Input: part model. Units: mm. Frame: model coordinates. Face numbers are marked on the shaded views. A direction names the side the tool comes from. Give positions to 0.01 mm unless a question says otherwise; leave off trailing zeros. Order: outer loops, then holes, each group sorted by start corner. A loop starts at its lowest first (then second) coordinate and runs counter-clockwise, first axis right, second up. Notation, with made-up numbers: (26.25, 72.25) - (82.25, 72.25) arc R24 cw to (82.25, 111.25) - close; hole circle Ø4 at (40.25, 83). An arc over 180 degrees is marked (long way). Use a Markdown table: item, result.
from build123d import *

# Parameters (mm, degrees)
F0_W        = 105
F0_H        = 23
F1_DEPTH    = 6.35
F2_W        = 72
F2_H        = 10
F3_DEPTH    = 25.4
F4_R        = 2.9337
F5_DEPTH    = 25.4
F6_T1_DEPTH = 6.35
F7_W        = 105
F7_H        = 23
F7_R        = 2.9335
F8_DEPTH    = 6.35
F9_W        = 72
F9_H        = 10
F10_DEPTH   = 25
F11_R       = 4.99999


# Not quite as in the source:
# - a fillet or chamfer that OpenCascade refuses, or shapes differently, is made with other operations: its cross-section is extruded or revolved along the edge and cut away or added
# - a fillet or chamfer is up to 0.001 mm smaller than in the source, because OpenCascade refuses the exact size


with BuildPart() as f1:
    # F0 (on Front) → F1 (new body)
    with BuildSketch(Plane.XZ):
        Rectangle(F0_W, F0_H)
    extrude(amount=F1_DEPTH)

    # F2 (on face) → F3 (cut)
    with BuildSketch(Plane.XZ.offset(6.35)):
        Rectangle(F2_W, F2_H)
    extrude(amount=-F3_DEPTH, mode=Mode.SUBTRACT)

    # F4 (on face) → F5 (cut)
    with BuildSketch(Plane.XZ.offset(6.35)):
        with Locations((-45, 0)):
            Circle(F4_R)
        with Locations((45, 0)):
            Circle(F4_R)
    extrude(amount=-F5_DEPTH, mode=Mode.SUBTRACT)

    # F6: fillet of radius 5.08 on 4 edges, made by hand

    # F6_s2 → F6_t1 (join)
    with BuildSketch(Plane.XZ):
        with BuildLine():
            ThreePointArc((36, 0.08), (34.5121024484, -3.5121024484), (30.92, -5))
            Line((30.92, -5), (36, -5))
            Line((36, -5), (36, 0.08))
        make_face()
        with BuildLine():
            ThreePointArc((-30.92, 5), (-34.5121024484, 3.5121024484), (-36, -0.08))
            Line((-36, -0.08), (-36, 5))
            Line((-36, 5), (-30.92, 5))
        make_face()
        with BuildLine():
            ThreePointArc((-30.92, -5), (-34.5121024484, -3.5121024484), (-36, 0.08))
            Line((-36, 0.08), (-36, -5))
            Line((-36, -5), (-30.92, -5))
        make_face()
        with BuildLine():
            ThreePointArc((36, -0.08), (34.5121024484, 3.5121024484), (30.92, 5))
            Line((30.92, 5), (36, 5))
            Line((36, 5), (36, -0.08))
        make_face()
    extrude(amount=F6_T1_DEPTH)

    # F7 (on Front) → F8 (join)
    with BuildSketch(Plane.XZ):
        with Locations((0, 22.8902743906)):
            Rectangle(F7_W, F7_H)
        with Locations((-45, 23.7624682486)):
            Circle(F7_R, mode=Mode.SUBTRACT)
        with Locations((45, 23.7624682486)):
            Circle(F7_R, mode=Mode.SUBTRACT)
    extrude(amount=F8_DEPTH)

    # F9 (on face) → F10 (cut)
    with BuildSketch(Plane.XZ.offset(6.35)):
        with Locations((0, 25.0778379703)):
            Rectangle(F9_W, F9_H)
    extrude(amount=-F10_DEPTH, mode=Mode.SUBTRACT)

    # F11 (radius 5 in the source; OpenCascade refuses exactly that, so slightly less here)
    f11_edges = [f1.edges().sort_by_distance(p)[0] for p in [
        (-36, -3.175, 20.077838),
        (36, -3.175, 20.077838),
        (36, -3.175, 30.077838),
        (-36, -3.175, 30.077838),
    ]]
    fillet(f11_edges, radius=F11_R)


solid = f1.part
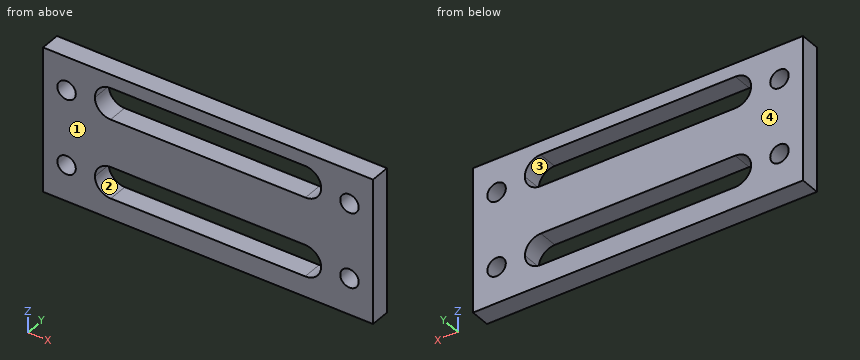
1. Material intervals for line 1 along Z through (x, y) = (45, -4.25); line 2 along Z through (x, y) = (-6, -6); line 3 along X through (y, z) = (-5.25, -2), sorted ascending.
Response:
| item | result |
|---|---|
| line 1 | z = -11.5 to -2.93, 2.93 to 20.83, 26.7 to 34.39 |
| line 2 | z = -11.5 to -5, 5 to 20.08, 30.08 to 34.39 |
| line 3 | x = -52.5 to -47.15, -42.85 to -35.55, 35.55 to 42.85, 47.15 to 52.5 |
2. Section query C-C (z = 1.5). Return loops of the section in (x, y).
Response:
| item | result |
|---|---|
| outline | (-52.5, -6.35) - (-47.52, -6.35) - (-47.52, 0) - (-52.5, 0) - close; (-42.48, -6.35) - (-35.75, -6.35) - (-35.75, 0) - (-42.48, 0) - close; (35.75, -6.35) - (42.48, -6.35) - (42.48, 0) - (35.75, 0) - close; (47.52, -6.35) - (52.5, -6.35) - (52.5, 0) - (47.52, 0) - close |
3. Mould query, pull axis Z, two halves, no side actions, for the marked faces 1 and 2. Classes: pulls with the +Z half, pulls with the -Z half, needs draft (parallel to the pull), parting line crosses it, or undercut.
Response:
| item | result |
|---|---|
| face 1 | needs draft |
| face 2 | undercut |
4. Set-up query: the marked faces 3 and 4. Return all of +Z, -Z, +X, -X, +Y, -Y with unobstructed straight access to the full face (end or side cutting, diameter ignored); none if empty.
Response:
| item | result |
|---|---|
| face 3 | +Y, -Y |
| face 4 | +Z, -Z, +X, -X, +Y |
5. Section query B-B (y = -2.5). State how many separate pieces and enclosed holes the cut face has, then the cut area to 3 significant figures.
Response:
| item | result |
|---|---|
| separate pieces | 1 |
| enclosed holes | 6 |
| area | 3,310 mm^2 |
6. Section query A-A (x = -6). Return loops of the section in (y, z), then the cut area to 3 significant figures.
Response:
| item | result |
|---|---|
| outline | (-6.35, -11.5) - (0, -11.5) - (0, -5) - (-6.35, -5) - close; (-6.35, 5) - (0, 5) - (0, 20.08) - (-6.35, 20.08) - close; (-6.35, 30.08) - (0, 30.08) - (0, 34.39) - (-6.35, 34.39) - close |
| area | 164 mm^2 |
7. Section query D-D (x = -45). Return loops of the section in (y, z).
Response:
| item | result |
|---|---|
| outline | (-6.35, -11.5) - (0, -11.5) - (0, -2.93) - (-6.35, -2.93) - close; (-6.35, 2.93) - (0, 2.93) - (0, 20.83) - (-6.35, 20.83) - close; (-6.35, 26.7) - (0, 26.7) - (0, 34.39) - (-6.35, 34.39) - close |
